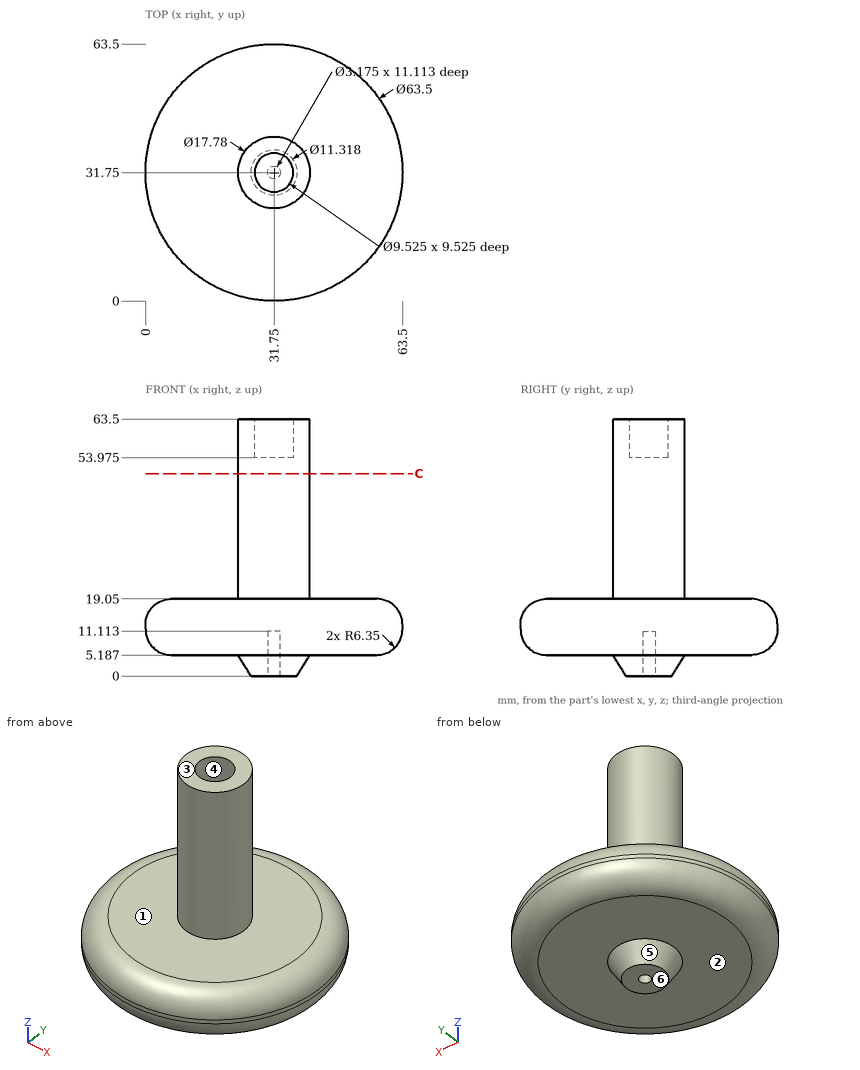
Geometry check sheet. Reference: drawing and pictorial views, mm from the part's lowest x, y, z. A direction names the side the tool comes from. Give positions to 0.01 mm unless a question says otherwise; leave off trailing zeros. Order: outer loops, then holes, each group sorted by start corner. A loop starts at its lowest first (then second) coordinate and runs counter-clockwise, first axis right, second up. Notation, with made-up numbers: M 64.25,16 L 99.25,16 A13 cw 99.25,20 Z; hole C -33.5,85.5 d8. An arc over 180 degrees is marked long. Answer in a Markdown table with one row per item. Add a question column.
Item 1: Scan lines: probe 1 along X at (y, z) = (31, 3); probe 2 along Z at (x, y) = (25, 46.5); probe 3 along Y at (x, z) = (31.75, 3.5). Record each from-to range of solid material in increasing order. Write a range as from..to.
Item 2: Gauge pin test, flat ends, axial feed: pin 1 (8.5 mm diameter, centred on x = 31.75, y = 31.75, fed in from +Z) (1 decimal); pin 2 (12 mm diameter, centred on x = 31, z = 23.5, fed in from -Y); pin 3 (12 mm diameter, centred on y = 12, z = 22, fed in from -X); pin 4 (8 mm diameter, centred on y = 45.5, z = 50.5, fed in from +X) (3 decimals). Record the tip position at first contact, or that the pin passes through.
Item 3: Tool access check on the marked faces 1, 2 and 3. Record the directions out of +Z, -Z, +X, -X, +Y, -Y that give a thin tool (end or side, any length) a straight path to the whole face; none if there is none.
Item 4: Mould release check, pull along Y, two halves, no side actions. Record for the marked faces 4, 5 and 6: released by +Y, released by -Y, zero draft, split by the parting line, or undercut.
Item 5: Section check C-C, the plane z = 50. Enter the section's corners in (x, y).
Filled sheet:
| question | item | result |
|---|---|---|
| 1 | probe 1 | x = 24.26..30.35, 33.15..39.24 |
| 1 | probe 2 | z = 5.19..19.05 |
| 1 | probe 3 | y = 23.91..30.16, 33.34..39.59 |
| 2 | pin 1 | stops at z = 54 |
| 2 | pin 2 | stops at y = 2.2 |
| 2 | pin 3 | stops at x = 6.56 |
| 2 | pin 4 | passes through |
| 3 | face 1 | +Z |
| 3 | face 2 | -Z |
| 3 | face 3 | +Z, +X, -X, +Y, -Y |
| 4 | face 4 | undercut |
| 4 | face 5 | split by the parting line |
| 4 | face 6 | zero draft |
| 5 | outline | C 31.75,31.75 d17.78 |
